from build123d import *

# Parameters (mm, degrees)
F0_W     = 320
F0_H     = 220
F0_R     = 2.5
F1_DEPTH = 6.2
F3_DEPTH = 3
F4_W     = 70
F4_H     = 20
F5_DEPTH = 25
F6_R     = 3


with BuildPart() as f1:
    # F0 (on Top) → F1 (new body)
    with BuildSketch(Plane.XY):
        Rectangle(F0_W, F0_H)
        with Locations((-154.5, -104.5)):
            Circle(F0_R, mode=Mode.SUBTRACT)
        with Locations((154.5, -104.5)):
            Circle(F0_R, mode=Mode.SUBTRACT)
        with Locations((-154.5, 104.5)):
            Circle(F0_R, mode=Mode.SUBTRACT)
        with Locations((154.5, 104.5)):
            Circle(F0_R, mode=Mode.SUBTRACT)
    extrude(amount=F1_DEPTH)

    # F2 (on face) → F3 (cut)
    with BuildSketch(Plane.XY.offset(6.2)):
        with BuildLine():
            Line((-15, 0), (15, 0))
            ThreePointArc((15, 0), (0, 15), (-15, 0))
        make_face()
        with BuildLine():
            Line((15, -110), (15, 0))
            ThreePointArc((15, 0), (0, -15), (-15, 0))
            Line((-15, 0), (-15, -110))
            Line((-15, -110), (15, -110))
        make_face()
        with BuildLine():
            ThreePointArc((-15, 0), (0, -15), (15, 0))
            Line((15, 0), (-15, 0))
        make_face()
    extrude(amount=-F3_DEPTH, mode=Mode.SUBTRACT)

    # F4 (on face) → F5 (cut)
    with BuildSketch(Plane.XY.offset(6.2)):
        with Locations((0, -100)):
            Rectangle(F4_W, F4_H)
    extrude(amount=-F5_DEPTH, mode=Mode.SUBTRACT)

    # F6
    f6_edges = [f1.edges().sort_by_distance(p)[0] for p in [
        (35, -90, 3.1),
        (-35, -90, 3.1),
    ]]
    fillet(f6_edges, radius=F6_R)


solid = f1.part
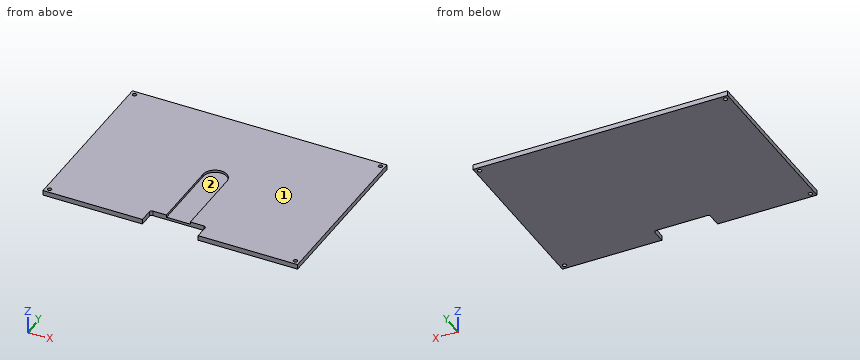
CAD build for the part. Positions are in the model's coordinates, mm. Face numbers are marked on the shaded views. Round coordinates to 2 decimals unless told otherwise and drop trailing zeros. Order: outer loops, then holes, each group sorted by start corner. A loop starts at its lowest first (then second) coordinate and runs counter-clockwise, first axis right, second up. Notation, with made-up numbers: M 67,-14.75 L 105,-14.75 A26 ccw 105,19.25 Z; hole C 60,32.25 d4. An arc over 180 degrees is marked long. Use one line per item in the form item = value.
Q1. Flat gauge pin, fed straight in: P1, Ø6, axis at x = 154.5, y = -104.5, coming from the -Z side. Where does the tip first touch, or does it go through?
Recorded:
P1 = 0
Q2. Saw through at A-A on y = -67. Give the cut face in (x, z).
Recorded:
outline = M -160,0 L 160,0 L 160,6.2 L 15,6.2 L 15,3.2 L -15,3.2 L -15,6.2 L -160,6.2 Z
Q3. Saw through at B-B on x = 0. Give the cut face in (y, z), then the cut area to 3 significant figures.
Recorded:
outline = M -90,0 L 110,0 L 110,6.2 L 15,6.2 L 15,3.2 L -90,3.2 Z
area = 925 mm^2
Q4. Probe L1, parallel to Y at x = -154.5, z = 3.25; L2, parallel to X at y = -29.5, z = 5; L3, parallel to X at y = -95.5, z = 2. List the from-to ranges inside material, lowest first.
Recorded:
L1 = -110 to -107, -102 to 102, 107 to 110
L2 = -160 to -15, 15 to 160
L3 = -160 to -35, 35 to 160
Q5. Two-plate mould, pull along X, no slides. Class the marked faces 1 and 2: +X half, -X half, draft (parallel to the pull), parting line (faces both ways), or undercut.
Recorded:
face_1 = draft
face_2 = undercut
